The figure shows three views and two pictorial views of one solid part (mm, origin at its lowest corner). Answer the questions. A direction names the side the tool comes from. Round coordinates to 2 decimals unless told otherwise and drop trailing zeros. Order: outer loops, then holes, each group sorted by start corner. A loop starts at its lowest first (then second) coordinate and runs counter-clockwise, first axis right, second up. Notation, with made-up numbers: (44.5, 40.5) -> (58.5, 40.5) arc R13 ccw to (58.5, 46.5) -> close; hole circle Ø4 at (-15.5, 50.5). An arc over 180 degrees is marked (long way). Answer as a JSON object with one key per item and string values. Group by question number.
Item 1: Consider probe 1 along X at (y, z) = (7.5, 5.25) (1 decimal); probe 2 along X at (y, z) = (5.75, 5) (1 decimal); probe 3 along Y at (x, z) = (10, 2.3). Determine where each line is inside the solid, lowest interval first. Write a range as from..to.
Item 2: Section C-C, the plane z = 6.75 is taken. Write down the section's boundary in (x, y) (1 decimal), plus the area to 3 significant figures.
Item 3: Given P1, Ø2, axis at y = 6, z = 5.5, coming from the +X side; P2, Ø5.5, axis at x = 21.72, y = 7.5, coming from the +Z side (1 decimal); P3, Ø6.5, axis at x = 90, y = 7.5, coming from the -Z side; P4, Ø7.5, axis at x = 12.5, y = 9.5, coming from the +Z side, each flat-ended and moving along its own axis, determine where each tip first touches the part or whether it passes through.
Item 4: Section A-A, the plane x = 10 is taken. Write down the section's boundary in (y, z).
Item 5: Section B-B, the plane y = 7.5 is taken. Count the separate pieces of the cut face and the enclosed holes in it, plus the area to 3 significant figures.
Item 6: Section D-D, the plane y = 3.5 is taken. Write down the section's boundary in (x, z), plus the area to 3 significant figures.
Item 7: For the marked faces 1, 2 and 3, determine the directions among +Z, -Z, +X, -X, +Y, -Y from which every point of the face is accessible in a straight line to the end or side of a thin tool.
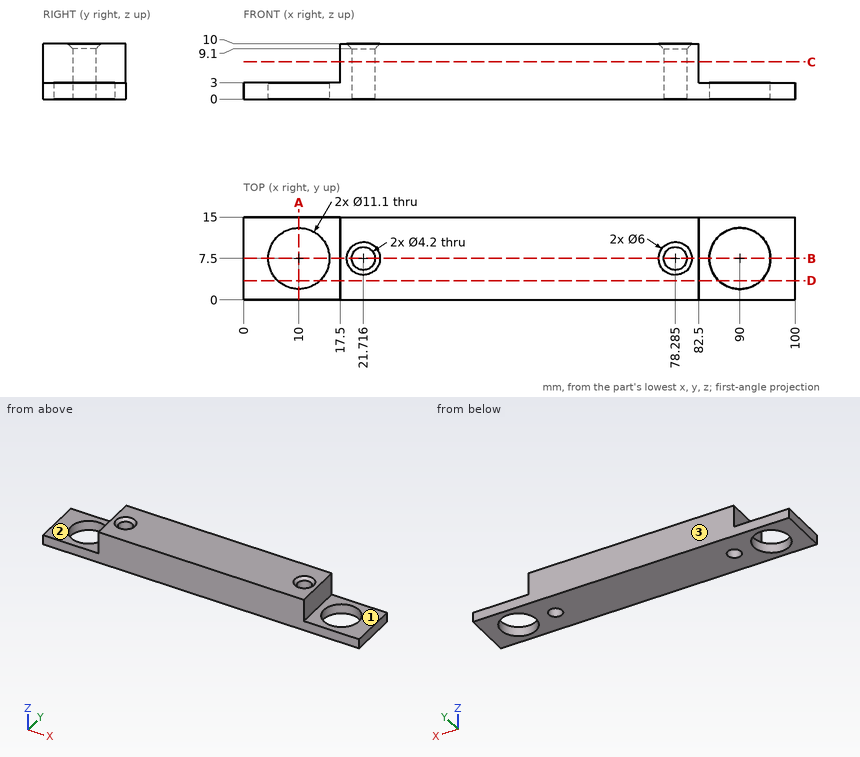
Values found:
{
 "1": {"probe 1": "17.5..19.6, 23.8..76.2, 80.4..82.5", "probe 2": "17.5..20.6, 22.9..77.1, 79.4..82.5", "probe 3": "0..1.95, 13.05..15"},
 "2": {"outline": "(17.5, 0) -> (82.5, 0) -> (82.5, 15) -> (17.5, 15) -> close; hole circle Ø4.2 at (21.7, 7.5); hole circle Ø4.2 at (78.3, 7.5)", "area": "947 mm2"},
 "3": {"P1": "x = 82.5", "P2": "z = 9.8", "P3": "through", "P4": "z = 3"},
 "4": {"outline": "(0, 0) -> (1.95, 0) -> (1.95, 3) -> (0, 3) -> close; (13.05, 0) -> (15, 0) -> (15, 3) -> (13.05, 3) -> close"},
 "5": {"separate pieces": "5", "enclosed holes": "0", "area": "603 mm2"},
 "6": {"outline": "(0, 0) -> (6.15, 0) -> (6.15, 3) -> (0, 3) -> close; (13.85, 0) -> (86.15, 0) -> (86.15, 3) -> (82.5, 3) -> (82.5, 10) -> (17.5, 10) -> (17.5, 3) -> (13.85, 3) -> close; (93.85, 0) -> (100, 0) -> (100, 3) -> (93.85, 3) -> close", "area": "709 mm2"},
 "7": {"face 1": "+Z, +X, +Y, -Y", "face 2": "+Z, -X, +Y, -Y", "face 3": "+Z, -Z, +X, -X, +Y"}
}
